Design review of the part built by this model. Coordinates are the model's own, in mm. A direction names the side the tool comes from. Coordinates: 2 decimals unless noted, no trailing zeros. Loops run counter-clockwise (first coordinate to the right, second up) from the corner with the lowest first, then second, coordinate; pieces in that order, holes last. Notation, with made-up numbers: (20, 48) -> (36, 48) arc R15 cw to (36, 56) -> close; hole circle Ø11 at (31.5, 88.25). An arc over 180 degrees is marked (long way). Answer as a JSON object with one key per item and string values.
```python
from build123d import *

# Parameters (mm, degrees)
SKETCH1_R           = 9.75
BOSS_EXTRUDE1_DEPTH = 5
SKETCH2_R           = 1.25
CUT_EXTRUDE1_DEPTH  = 5
CHAMFER1_SIZE       = 2.5
SKETCH4_R           = 2.5
CUT_EXTRUDE3_DEPTH  = 2.5


with BuildPart() as part:
    # Sketch1 → Boss-Extrude1 (new body)
    with BuildSketch(Plane.XY):
        Circle(SKETCH1_R)
    extrude(amount=BOSS_EXTRUDE1_DEPTH)

    # Sketch2 → Cut-Extrude1 (cut)
    with BuildSketch(Plane(origin=(0, 0, 0), x_dir=(-1, 0, 0), z_dir=(0, 0, -1))):
        Circle(SKETCH2_R)
    extrude(amount=-CUT_EXTRUDE1_DEPTH, mode=Mode.SUBTRACT)

    # Chamfer1
    chamfer1_edges = [part.edges().sort_by_distance(p)[0] for p in [
        (-9.75, 0, 5),
    ]]
    chamfer(chamfer1_edges, length=CHAMFER1_SIZE)

    # Sketch4 → Cut-Extrude3 (cut)
    with BuildSketch(Plane(origin=(0, 0, 0), x_dir=(-1, 0, 0), z_dir=(0, 0, -1))):
        Circle(SKETCH4_R)
    extrude(amount=-CUT_EXTRUDE3_DEPTH, mode=Mode.SUBTRACT)


solid = part.part
```
1) Wall thickness on probe 1 along Y at (x, z) = (0, 1.5); probe 2 along Y at (x, z) = (0, 3.35); probe 3 along X at (y, z) = (-1, 2): over which ranges is each line inside the solid? List them lowest first.
Completed:
{"probe 1": "-9.75 to -2.5, 2.5 to 9.75", "probe 2": "-8.9 to -1.25, 1.25 to 8.9", "probe 3": "-9.7 to -2.29, 2.29 to 9.7"}
2) Add section C-C, the plane z = 1.9. Give the boundary of the cut face in (x, y), and give its area (3 significant figures).
Completed:
{"outline": "circle Ø19.5 at (0, 0); hole circle Ø5 at (0, 0)", "area": "279 mm²"}
3) Add section A-A, the plane y = 0. Give the boundary of the cut face in (x, z), and give its area (3 significant figures).
Completed:
{"outline": "(-9.75, 0) -> (-2.5, 0) -> (-2.5, 2.5) -> (-1.25, 2.5) -> (-1.25, 5) -> (-7.25, 5) -> (-9.75, 2.5) -> close; (1.25, 2.5) -> (2.5, 2.5) -> (2.5, 0) -> (9.75, 0) -> (9.75, 2.5) -> (7.25, 5) -> (1.25, 5) -> close", "area": "72.5 mm²"}
4) Add section D-D, the plane z = 3.35. Give the boundary of the cut face in (x, y), and give its area (3 significant figures).
Completed:
{"outline": "circle Ø17.8 at (0, 0); hole circle Ø2.5 at (0, 0)", "area": "244 mm²"}
5) For faces 4 (the flat face through (2, -2, 0)), 5 (the flat face through (1, -1, 2.5)), list the 3-axis set-ups (+Z, -Z, +X, -X, +Y, -Y) from which the entire face can be reached by the end or side of a thin tool; tool diameter is ignored.
Completed:
{"face 4": "-Z, +X, -X, +Y, -Y", "face 5": "-Z"}
6) Clearance check with flat-ended pins moving along their axes: pin 1 Ø2 at (x, z) = (6, 1.5) entering from -Y; pin 2 Ø3 at (y, z) = (-5.5, 1) entering from -X; pin 3 Ø1.5 at (y, z) = (-4.5, 3.5) entering from +X. State where each tip first meets the part, or that it passes through.
Completed:
{"pin 1": "y = -8.37", "pin 2": "x = -8.89", "pin 3": "x = 8.45"}
7) The part is to be moulded in two halves that separate along X. For faces 1 (the flat face through (2, 0, 5)), 2 (the cylindrical face through (0.27, -1.22, 3.73)), 3 (the cylindrical face through (-1.269, 9.667, 1.232)), say which applies: pulls with the +X half, pulls with the -X half, needs draft (parallel to the pull), parting line crosses it, or undercut.
Completed:
{"face 1": "needs draft", "face 2": "undercut", "face 3": "parting line crosses it"}
